Model file for the job. Use its own axes, mm. A direction names the side the tool comes from. Round coordinates to 2 decimals unless told otherwise and drop trailing zeros. Order: outer loops, then holes, each group sorted by start corner. A loop starts at its lowest first (then second) coordinate and runs counter-clockwise, first axis right, second up. Notation, with made-up numbers: (-32.5, -16) -> (25.5, -16) arc R28 cw to (25.5, 19) -> close; hole circle Ø6 at (-15, 89). An arc over 180 degrees is marked (long way). Put each result on its own line as item: value. Start each with the question number.
Q1. Cut at A-A, the plane x = 17. List the corners of the cut face in (y, z), and give its area (3 significant figures).
Q2. Pull direction Z, two halves, no side cores. Call faces 1 (the face through (9.392, -2.348, -4.144)), 2 (the face through (9.653, 2.208, 1.149)), 3 (the face through (9.39, -2.41, 4.11)): released by +Z, released by -Z, zero draft, split by the parting line, or undercut.
Q3. Flat gauge pin, fed straight in: P1, Ø3, axis at x = 15, y = -2.5, coming from the -Z side. Where does the tip first touch, or does it go through?
Q4. 3-axis set-ups, long thin cutter, end or side, ignore diameter. For faces 4 (the face through (18.966, 0.012, -4.942)), 5 (the face through (9.649, -3.514, 0.944)): which of +Z, -Z, +X, -X, +Y, -Y reach the whole face in a straight line?
Q5. Probe L1, parallel to X at y = -3.65, z = 0; L2, parallel to Z at x = 2.5, y = -1; L3, parallel to Z at x = 12, y = -1.25. List the from-to ranges inside material, lowest first.
Q6. Cut at B-B, the plane z = -0.5. State how many separate pieces and enclosed holes the cut face has, and give its area (3 significant figures).
Autodesk Inventor part; units mm, degrees
ref_plane "Work Plane1" through (23.9707, 0, 0) normal (0, 1, 0) x (-1, 0, 0)
ref_plane "YZ Plane" through (0, 0, 0) normal (1, 0, 0) x (0, 1, 0)
ref_plane "XZ Plane" through (0, 0, 0) normal (0, 1, 0) x (-1, 0, 0)
sketch "Sketch1" plane through (0, 0, 0) normal (1, 0, 0) x (0, 1, 0)
  line L0 (-6.6675, 0) -> (6.6675, 0)
  line L1 (0, -7.699) -> (0, 7.699)
  line L2 (0, 5.4993) -> (4.7625, 2.7496)
  line L3 (4.7625, 2.7496) -> (4.7625, -2.7496)
  line L4 (4.7625, -2.7496) -> (0, -5.4993)
  line L5 (0, -5.4993) -> (-4.7625, -2.7496)
  line L6 (-4.7625, -2.7496) -> (-4.7625, 2.7496)
  line L7 (-4.7625, 2.7496) -> (0, 5.4993)
  point P0 (0, 0)
  dimension "d40" = 9.525
extrude "Body" add sketch "Sketch1" along normal blind 19.05
sketch "Sketch2" plane through (0, 0, 0) normal (-1, 0, 0) x (0, 0, 1)
  line L0 (0, -6.6675) -> (0, 6.6675)
  line L1 (-7.699, 0) -> (7.699, 0)
  point P0 (0, 0)
hole "Thread" at (0, 0, 0) direction (1, 0, 0) diameter 4.9784 end through all
sketch "Sketch3" plane through (0, 0, 0) normal (0, 0, 1) x (1, 0, 0)
  line L0 (-3.81, 0) -> (22.86, 0)
  line L1 (0, 0) -> (0, 4.7625)
  line L2 (19.05, 0) -> (19.05, 4.7625)
  line L3 (0, 4.7625) -> (19.05, 4.7625) construction
  line L4 (0, 5.4993) -> (0, 4.7625)
  line L5 (0, 4.7625) -> (0.3436, 5.4993)
  line L6 (0.3436, 5.4993) -> (0, 5.4993)
  line L7 (19.05, 4.7625) -> (19.05, 5.4993)
  line L8 (19.05, 5.4993) -> (18.7064, 5.4993)
  line L9 (18.7064, 5.4993) -> (19.05, 4.7625)
  line L10 (0.3436, 5.4993) -> (18.7064, 5.4993)
  line L11 (0, 4.7625) -> (19.05, 4.7625)
  line L12 (0, 0) -> (19.05, 0)
  dimension "d45" = 9.525
  dimension "d46" = 10.9985
  dimension "d47" = 25
  dimension "d48" = 25
revolve "Chamfer1" cut sketch "Sketch3" angle 360 about axis through (-10, 0, 0) along (1, 0, 0) contours L4 L6 L5 | L9 L8 L7
chamfer "Chamfer2" distance 0.6874 angle 30 1 edges at (0, 0, -2.4892) measured on face at (0, 2.8968, -2.7339)
chamfer "Chamfer3" distance 0.6874 angle 30 1 edges at (19.05, 0, -2.4892) measured on face at (19.05, 2.8968, -2.7339)
sketch "Sketch4" plane through (0, 0, 0) normal (0, 1, 0) x (-1, 0, 0)
  line L0 (0, -1.3335) -> (0, 1.3335)
  line L1 (-8.1915, 0) -> (-10.8585, 0)
  circle A0 centre (-9.525, 0) radius 0.9525
  dimension "d36" = 1.905
  dimension "d37" = 9.525
extrude "Hole" cut sketch "Sketch4" against normal through all
ref_plane "Work Plane1" through (23.9707, 0, 0) normal (0, 1, 0) x (-1, 0, 0)
equation "\"d40\" = SW"
equation "\"d1\" = KOH"
equation "\"d8\" = -0.5 * GD1 + 0.5 * NND"
equation "\"d49\" = -0.5 * GD1 + 0.5 * NND"
equation "\"d10\" = -0.5 * GD1 + 0.5 * NND"
equation "\"d50\" = -0.5 * GD1 + 0.5 * NND"
equation "\"d36\" = BOR"
equation "\"d37\" = 0.5 * KOH"
equation "\"d45\" = SW0"
equation "\"d46\" = 1.1547 * SW"
equation "\"d47\" = ANG1"
equation "\"d48\" = ANG2"
equation "\"ANG1\" = 25deg"
equation "\"ANG2\" = 25deg"
equation "\"NND\" = 6.35"
equation "\"KOH\" = 19.05"
equation "\"SW\" = 9.525"
equation "\"SW0\" = SW"
equation "\"SW01\" = SW"
equation "\"BOR\" = 1.905"
equation "\"THREADDIA\" = 6.35"
equation "\"TOA\" = 30deg"
equation "\"DIST\" = 0.5 * KOH"
equation "\"E0\" = 1.155 * SW"
properties part number "IFI 128 - 1/4 - 20" material "Steel, Mild"
Ans:
1. outline: (-4.76, -2.75) -> (0, -5.5) -> (4.76, -2.75) -> (4.76, 2.75) -> (0, 5.5) -> (-4.76, 2.75) -> close; hole circle Ø4.98 at (0, 0)
1. area: 59.1 mm^2
2. face 1: released by -Z
2. face 2: undercut
2. face 3: released by +Z
3. P1: stops at z = -4.92
4. face 4: -Z, +X
4. face 5: -Y
5. L1: x = 0 to 8.57, 10.48 to 19.05
5. L2: z = -4.92 to -2.28, 2.28 to 4.92
5. L3: z = -4.78 to -2.15, 2.15 to 4.78
6. separate pieces: 3
6. enclosed holes: 0
6. area: 84.2 mm^2
